The figure shows three views and two pictorial views of one solid part (mm, origin at its lowest corner). Answer the questions. A direction names the side the tool comes from. Round coordinates to 2 decimals unless told otherwise and drop trailing zeros. Write each loop counter-clockwise with the first axis right and the second up, starting at its lowest first coordinate (ties: lowest second). Pieces come first, ordered by that corner, then holes. Notation, with made-up numbers: (67, 9.5) -> (90, 9.5) arc R20 ccw to (90, 22.5) -> close; hole circle Ø3 at (32, 14.5). An arc over 180 degrees is marked (long way). One line per item, written item: value.
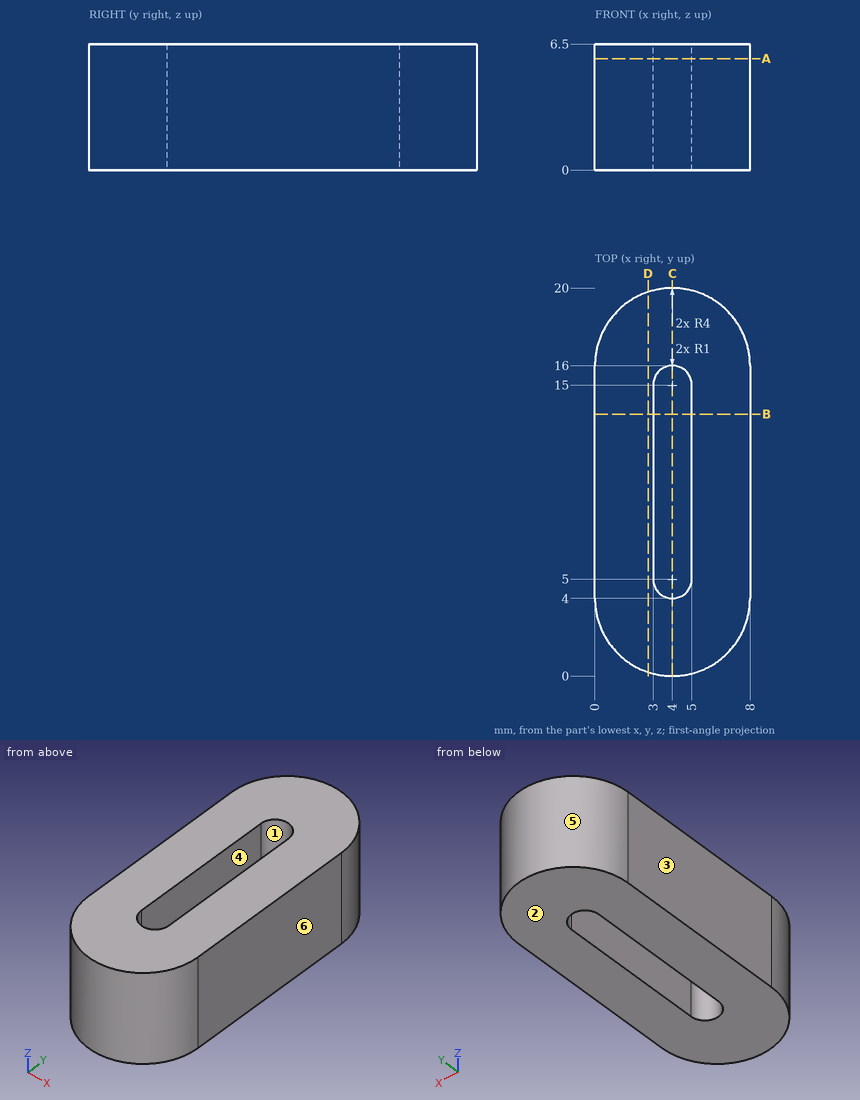
(1) Find section D-D on x = 2.75. Give the vertices of the cut face in (y, z).
Reported:
outline: (0.2, 0) -> (19.8, 0) -> (19.8, 6.5) -> (0.2, 6.5) -> close
(2) Consider probe 1 along X at (y, z) = (9.75, 2); probe 2 along Y at (x, z) = (4, 4.75); probe 3 along X at (y, z) = (4.25, 4.75). Determine where each line is inside the solid, lowest interval first.
Reported:
probe 1: x = 0 to 3, 5 to 8
probe 2: y = 0 to 4, 16 to 20
probe 3: x = 0 to 3.34, 4.66 to 8
(3) Find section B-B on y = 13.5. Give the vertices of the cut face in (x, z), plus the area to 3 significant figures.
Reported:
outline: (0, 0) -> (3, 0) -> (3, 6.5) -> (0, 6.5) -> close; (5, 0) -> (8, 0) -> (8, 6.5) -> (5, 6.5) -> close
area: 39.0 mm2
(4) Find section A-A on z = 5.75. Give the vertices of the cut face in (x, y), plus the area to 3 significant figures.
Reported:
outline: (0, 4) arc R4 ccw to (8, 4) -> (8, 16) arc R4 ccw to (0, 16) -> close; hole (3, 5) arc R1 ccw to (5, 5) -> (5, 15) arc R1 ccw to (3, 15) -> close
area: 123 mm2
(5) Find section C-C on x = 4. Give the vertices of the cut face in (y, z).
Reported:
outline: (0, 0) -> (4, 0) -> (4, 6.5) -> (0, 6.5) -> close; (16, 0) -> (20, 0) -> (20, 6.5) -> (16, 6.5) -> close
(6) For a pull along X with two mould halves and no side action, classify the marked faces 3, 4, 5 and 6 as pulls with the +X half, pulls with the -X half, needs draft (parallel to the pull), parting line crosses it, or undercut.
Reported:
face 3: pulls with the -X half
face 4: undercut
face 5: parting line crosses it
face 6: pulls with the +X half
(7) A tool of negligible diameter and unlimited length cuts with its end or side. For the marked faces 1 and 2, from which of +Z, -Z, +X, -X, +Y, -Y can it reach the whole face along a straight path? Write none if from no direction.
Reported:
face 1: +Z, -Z
face 2: -Z, +X, -X, +Y, -Y
